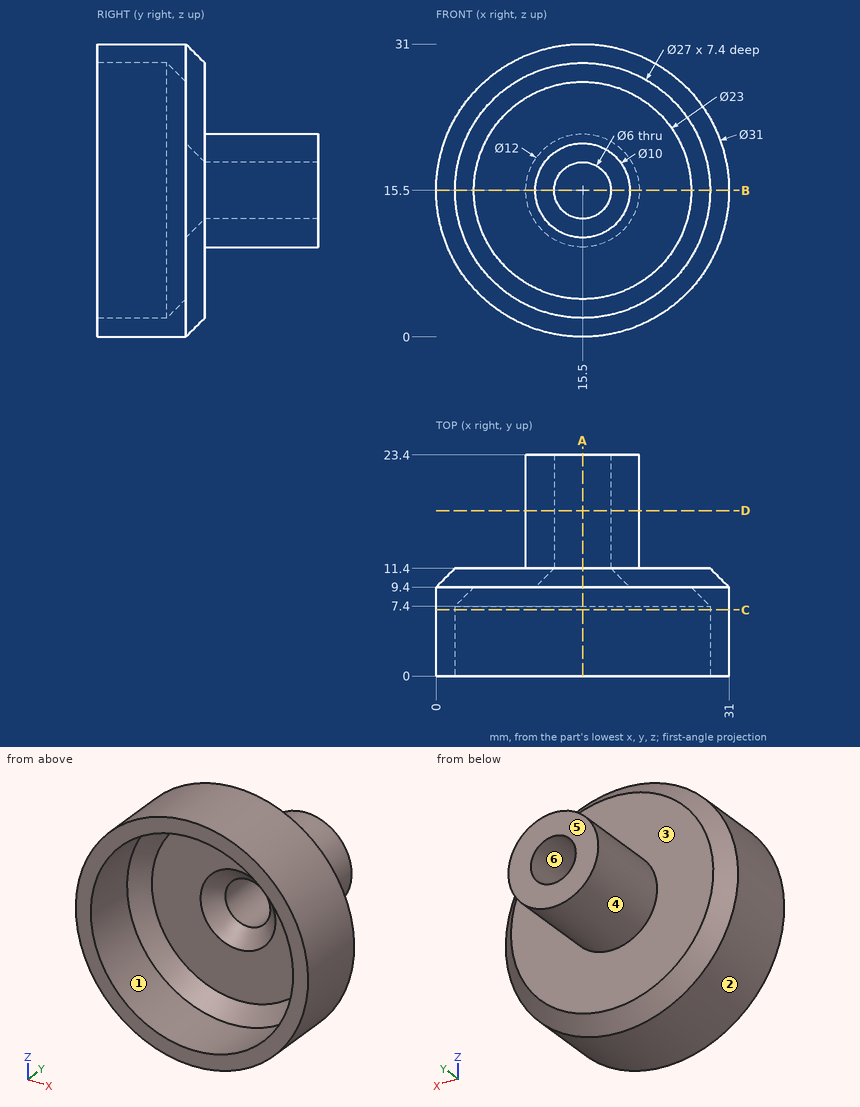
Geometry check sheet. Reference: drawing and pictorial views, mm from the part's lowest x, y, z. A direction names the side the tool comes from. Give positions to 0.01 mm unless a question says otherwise; leave off trailing zeros. Order: outer loops, then holes, each group sorted by start corner. A loop starts at its lowest first (then second) coordinate and runs counter-clockwise, first axis right, second up.
1. Section check C-C, the plane y = 7. Enter the section's corners in (x, z), and give its area (3 significant figures).
2. Access from +Z, -Z, +X, -X, +Y, -Y to the whole of each face (thin tool, end or side, straight path). Record for the marked faces 1, 2 and 3.
3. Section check D-D, the plane y = 17.5. Enter the section's corners in (x, z).
4. Section check A-A, the plane x = 15.5. Enter the section's corners in (y, z).
5. Release check for a two-part mould opening along X. For the marked faces 4, 5 and 6 record: pulls with the +X half, pulls with the -X half, needs draft (parallel to the pull), parting line crosses it, or undercut.
6. Thickness scan on L1, parallel to X at y = 15.5, z = 15.5; L2, parallel to X at y = 2.5, z = 15.5; L3, parallel to Y at x = 5.5, z = 10. Record the ranges inside material, lowest first.
7. Gauge pin test, flat ends, axial feed: pin 1 Ø5 at (x, y) = (24.5, 13) entering from -Z; pin 2 Ø3 at (x, y) = (3.5, 13.5) entering from -Z; pin 3 Ø2 at (x, z) = (3, 11.5) entering from +Y; pin 4 Ø8 at (y, z) = (19.5, 10) entering from -X. Record the tip position at first contact, or that the pin passes through.
8. Section check B-B, the plane z = 15.5. Enter the section's corners in (x, y).
Values follow:
1. outline: circle Ø31 at (15.5, 15.5); hole circle Ø27 at (15.5, 15.5)
1. area: 182 mm2
2. face 1: -Y
2. face 2: +Y, -Y
2. face 3: +Y
3. outline: circle Ø12 at (15.5, 15.5); hole circle Ø6 at (15.5, 15.5)
4. outline: (0, 0) - (9.4, 0) - (11.4, 2) - (11.4, 9.5) - (23.4, 9.5) - (23.4, 12.5) - (11.4, 12.5) - (9.4, 10.5) - (9.4, 4) - (7.4, 2) - (0, 2) - close; (0, 29) - (7.4, 29) - (9.4, 27) - (9.4, 20.5) - (11.4, 18.5) - (23.4, 18.5) - (23.4, 21.5) - (11.4, 21.5) - (11.4, 29) - (9.4, 31) - (0, 31) - close
5. face 4: parting line crosses it
5. face 5: needs draft
5. face 6: undercut
6. L1: x = 9.5 to 12.5, 18.5 to 21.5
6. L2: x = 0 to 2, 29 to 31
6. L3: y = 9.4 to 11.4
7. pin 1: stops at z = 3.76
7. pin 2: passes through
7. pin 3: stops at y = 11.4
7. pin 4: stops at x = 9.69
8. outline: (0, 0) - (2, 0) - (2, 7.4) - (4, 9.4) - (10.5, 9.4) - (12.5, 11.4) - (12.5, 23.4) - (9.5, 23.4) - (9.5, 11.4) - (2, 11.4) - (0, 9.4) - close; (18.5, 11.4) - (20.5, 9.4) - (27, 9.4) - (29, 7.4) - (29, 0) - (31, 0) - (31, 9.4) - (29, 11.4) - (21.5, 11.4) - (21.5, 23.4) - (18.5, 23.4) - close
